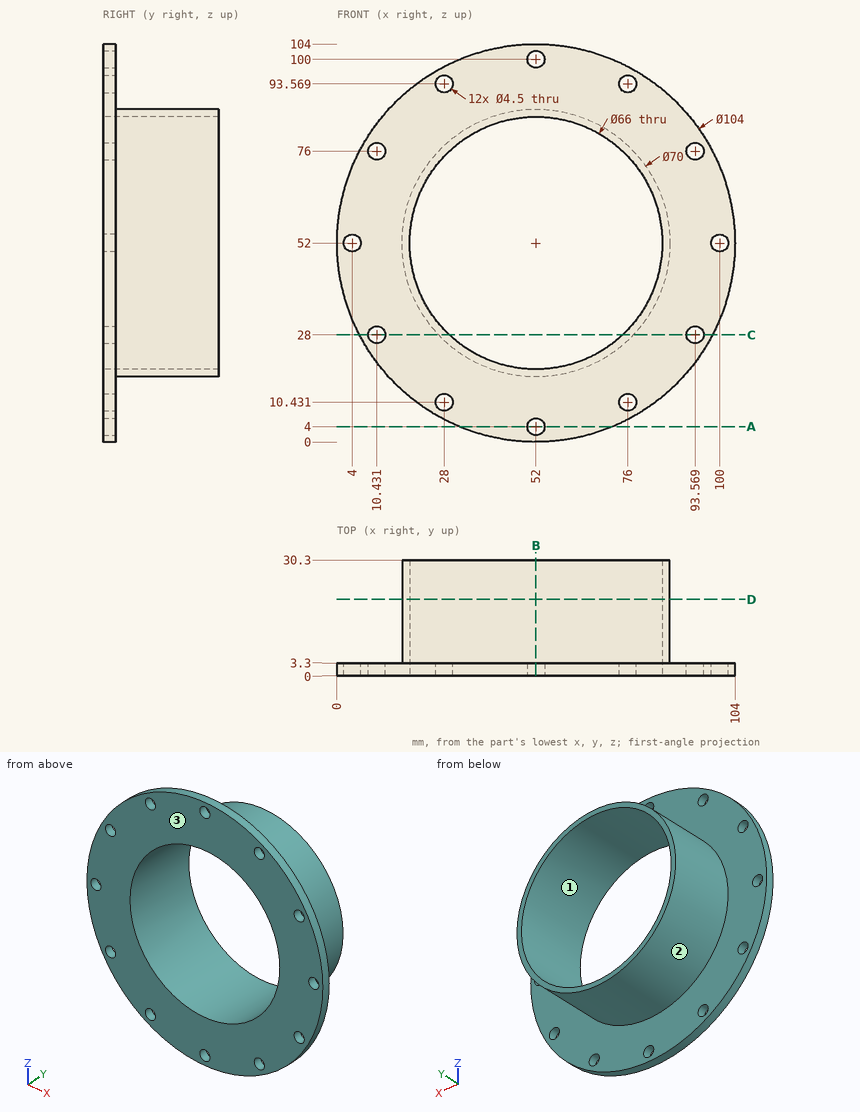
Source: three-view drawing plus pictorial views. Frame: mm from the lowest corner of the part. Coordinates: 2 decimals unless noted, no trailing zeros. Loops run counter-clockwise (first coordinate to the right, second up) from the corner with the lowest first, then second, coordinate; pieces in that order, holes last. Notation, with made-up numbers: (59.5, 21) -> (72.5, 21) arc R30 ccw to (72.5, 52) -> close; hole circle Ø1 at (70.25, -36.5). An arc over 180 degrees is marked (long way). One line per item, written item: value.
(1) Cut plane C-C (z = 28). Output: boundary loops of the cut face in (x, y).
Answer below:
outline: (5.87, 0) -> (8.18, 0) -> (8.18, 3.3) -> (5.87, 3.3) -> close; (12.68, 0) -> (29.35, 0) -> (29.35, 30.3) -> (26.52, 30.3) -> (26.52, 3.3) -> (12.68, 3.3) -> close; (74.65, 0) -> (91.32, 0) -> (91.32, 3.3) -> (77.48, 3.3) -> (77.48, 30.3) -> (74.65, 30.3) -> close; (95.82, 0) -> (98.13, 0) -> (98.13, 3.3) -> (95.82, 3.3) -> close
(2) Cut plane A-A (z = 4). Output: boundary loops of the cut face in (x, y), then the cut area to 3 significant figures.
Answer below:
outline: (32, 0) -> (49.75, 0) -> (49.75, 3.3) -> (32, 3.3) -> close; (54.25, 0) -> (72, 0) -> (72, 3.3) -> (54.25, 3.3) -> close
area: 117 mm2
(3) Pin query (flat end, axial travel): pin 1 Ø7 at (x, z) = (28, 93.57) entering from -Y; pin 2 Ø5 at (x, z) = (4, 52) entering from +Y; pin 3 Ø3 at (x, y) = (36, 20) entering from -Z (1 decimal); pin 4 Ø3 at (y, z) = (5.5, 51.5) entering from -X. Return the tip coordinate at first contact, or that it passes through.
Answer below:
pin 1: stops at y = 0
pin 2: stops at y = 3.3
pin 3: stops at z = 20.1
pin 4: stops at x = 17
(4) Cut plane D-D (y = 20). Output: boundary loops of the cut face in (x, z).
Answer below:
outline: circle Ø70 at (52, 52); hole circle Ø66 at (52, 52)
(5) Draft query along X for the marked faces 1, 2 and 3. Return one class per face: pulls with the +X half, pulls with the -X half, needs draft (parallel to the pull), parting line crosses it, or undercut.
Answer below:
face 1: undercut
face 2: parting line crosses it
face 3: needs draft
(6) Cut plane B-B (x = 52). Output: boundary loops of the cut face in (y, z).
Answer below:
outline: (0, 0) -> (3.3, 0) -> (3.3, 1.75) -> (0, 1.75) -> close; (0, 6.25) -> (3.3, 6.25) -> (3.3, 17) -> (30.3, 17) -> (30.3, 19) -> (0, 19) -> close; (0, 85) -> (30.3, 85) -> (30.3, 87) -> (3.3, 87) -> (3.3, 97.75) -> (0, 97.75) -> close; (0, 102.25) -> (3.3, 102.25) -> (3.3, 104) -> (0, 104) -> close
(7) Ray query, line 1 along X through (y, z) = (2, 28); line 2 along Z through (x, y) = (52, 9); line 3 along Y through (x, z) = (15, 70.5). Return the intervals inside material, ascending.
Answer below:
line 1: x = 5.87 to 8.18, 12.68 to 29.35, 74.65 to 91.32, 95.82 to 98.13
line 2: z = 17 to 19, 85 to 87
line 3: y = 0 to 3.3
